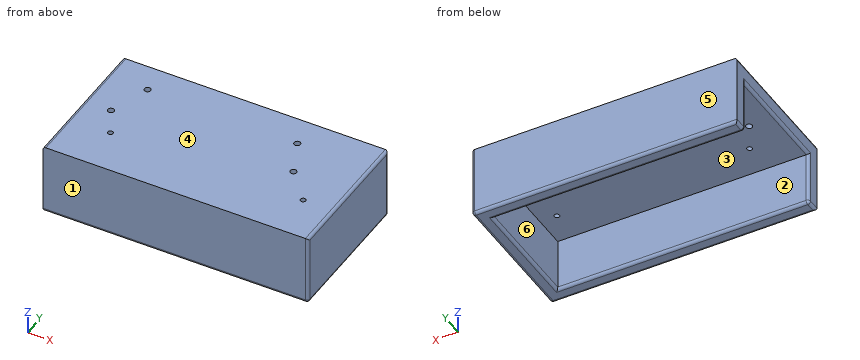
Autodesk Inventor part; units mm, degrees
ref_plane "YZ Plane" through (0, 0, 0) normal (1, 0, 0) x (0, 1, 0)
ref_plane "XZ Plane" through (0, 0, 0) normal (0, 1, 0) x (-1, 0, 0)
ref_plane "XY Plane" through (0, 0, 0) normal (0, 0, 1) x (1, 0, 0)
sketch "스케치1" plane through (0, 0, 0) normal (0, 0, 1) x (1, 0, 0)
  line L0 (-50.4495, 22.5) -> (42.4495, 22.5)
  line L1 (42.4495, 22.5) -> (42.4495, -27.5)
  line L2 (42.4495, -27.5) -> (-50.4495, -27.5)
  line L3 (-50.4495, -27.5) -> (-50.4495, 22.5)
  line L4 (-50.4495, 17.5) -> (37.5505, 17.5)
  line L5 (37.5505, 17.5) -> (37.5505, -22.5)
  line L6 (37.5505, -22.5) -> (-50.4495, -22.5)
  point P0 (0, 0)
  dimension "d0" = 40
  dimension "d1" = 88
  dimension "d2" = 5
  dimension "d3" = 5
extrude "돌출1" add sketch "스케치1" against normal blind 6.2 contours L4 L5 L6 L3
extrude "돌출2" add sketch "스케치1" against normal blind 25 contours L0 L1 L2 L3 L6 L5 L4
sketch "스케치2" plane through (0, 0, -6.2) normal (0, 0, -1) x (-1, 0, 0)
  circle A0 centre (36.2565, 12.6083) radius 1.1
  circle A1 centre (-16.5389, 11.9083) radius 1.1
  circle A2 centre (41.0611, -1.7917) radius 1.1
  circle A3 centre (-22.2389, -0.6917) radius 1.1
  circle A4 centre (35.8561, -11.3917) radius 0.9
  circle A5 centre (-31.6439, -11.3917) radius 0.9
  point P0 (0, 0)
  dimension "d8" = 52.8
  dimension "d9" = 2.2
  dimension "d10" = 2.2
  dimension "d11" = 2.2
  dimension "d12" = 2.2
  dimension "d13" = 63.3
  dimension "d14" = 14.4
  dimension "d15" = 12.6
  dimension "d16" = 1.8
  dimension "d17" = 1.8
  dimension "d18" = 67.5
  dimension "d19" = 10.7
  dimension "d23" = 9.405
  dimension "d24" = 0
  dimension "d25" = 0.7
  dimension "d26" = 5.7
extrude "돌출3" cut sketch "스케치2" against normal blind 63.3
sketch "스케치3" plane through (42.4495, -27.5, 0) normal (1, 0, 0) x (0, 0, -1)
  line L0 (-14.75, 0) -> (-14.75, 50)
  line L1 (-14.75, 50) -> (39.75, 50)
  line L2 (39.75, 50) -> (39.75, 0)
  line L3 (39.75, 0) -> (-14.75, 0)
  line L4 (0, 0) -> (0, 50)
  line L5 (-9.15, 0) -> (-9.15, 50)
  line L6 (34.15, 0) -> (34.15, 50)
  point P0 (0, 27.5)
  dimension "d27" = 54.5
  dimension "d28" = 14.75
  dimension "d29" = 5.6
  dimension "d30" = 43.3
extrude "돌출4" add sketch "스케치3" along normal blind 10
extrude "돌출5" add sketch "스케치3" along normal blind 80 contours L0 L1 L5 L3 | L6 L1 L2 L3
sketch "스케치4" plane through (42.4495, -27.5, 14.75) normal (0, 0, 1) x (1, 0, 0)
  circle A0 centre (25, 27.5) radius 3.75
  line L0 (0, 50) -> (0, 0)
  point P0 (-42.4495, 27.5)
  dimension "d35" = 7.5
  dimension "d36" = 25
extrude "돌출6" cut sketch "스케치4" against normal blind 80
ref_plane "작업 평면1" through (42.4495, -27.5, 0) normal (-1, 0, 0) x (0, 0, 1)
split "분할1" plane through (42.4495, -27.5, 0) removes the side toward (1, 0, 0)
sketch "스케치5" plane through (42.4495, -27.5, 0) normal (1, 0, 0) x (0, 0, -1)
  point P0 (0, 27.5)
sketch "스케치6" plane through (42.4495, -27.5, 0) normal (1, 0, 0) x (0, 0, -1)
  point P0 (0, 27.5)
fillet "모깎기2" radius 1 15 edges at (-6.4495, -22.5, -25) (37.5505, -2.5, -25) (-6.4495, 17.5, -25) (-4, 22.5, -25) (-50.4495, 20, -25) (-50.4495, -25, -25) (-4, -27.5, -25) (42.4495, -2.5, -25) (42.4495, -2.5, 0) (-50.4495, -2.5, 0) (-50.4495, -2.5, -6.2) (-50.4495, 17.5, -15.6) (-50.4495, -22.5, -15.6) (42.4495, 22.5, -12.5) (42.4495, -27.5, -12.5)
equation "\"d21\" = d13"
properties part number "Camera Housing Camera2"
Check sheet for the modelled part. Datum: model origin and axes. Units: mm. Face numbers are marked on the shaded views. A direction names the side the tool comes from. Give positions to 0.01 mm unless a question says otherwise; leave off trailing zeros. Write each loop counter-clockwise with the first axis right and the second up, starting at its lowest first coordinate (ties: lowest second). Pieces come first, ordered by that corner, then holes. Notation, with made-up numbers: M 17,-13 L 45,-13 A18 cw 45,8 Z; hole C 14,-20.75 d5. An arc over 180 degrees is marked long. Use one line per item in the form item = value.
(1) Section check C-C on y = -19. Record the boundary of the cut face in (x, z), plus the area to 3 significant figures.
Answer block:
outline = M -50.45,-5.2 A1 ccw -49.45,-6.2 L 37.55,-6.2 L 37.55,-24 A1 ccw 38.55,-25 L 41.45,-25 A1 ccw 42.45,-24 L 42.45,-1 A1 ccw 41.45,0 L -49.45,0 A1 ccw -50.45,-1 Z
area = 667 mm2
(2) Tool access check on the marked faces 5 and 6. Record the directions out of +Z, -Z, +X, -X, +Y, -Y that give a thin tool (end or side, any length) a straight path to the whole face; none if there is none.
Answer block:
face_5 = +Z, -Z, +X, -X, +Y
face_6 = -Z, -X
(3) Section check B-B on x = -24. Record the boundary of the cut face in (y, z), plus the area to 3 significant figures.
Answer block:
outline = M -27.5,-24 A1 ccw -26.5,-25 L -23.5,-25 A1 ccw -22.5,-24 L -22.5,-6.2 L 17.5,-6.2 L 17.5,-24 A1 ccw 18.5,-25 L 21.5,-25 A1 ccw 22.5,-24 L 22.5,0 L -27.5,0 Z
area = 497 mm2
(4) Draft check along Y on the marked faces 1, 2, 3 and 4. Enter one of: pulls with the +Y half, pulls with the -Y half, needs draft (parallel to the pull), parting line crosses it, or undercut.
Answer block:
face_1 = pulls with the -Y half
face_2 = undercut
face_3 = undercut
face_4 = needs draft
(5) Section check A-A on z = -22.75. Record the boundary of the cut face in (x, y).
Answer block:
outline = M -50.45,-27.5 L 41.45,-27.5 A1 ccw 42.45,-26.5 L 42.45,21.5 A1 ccw 41.45,22.5 L -50.45,22.5 L -50.45,18.5 A1 ccw -49.45,17.5 L 37.55,17.5 L 37.55,-22.5 L -49.45,-22.5 A1 ccw -50.45,-23.5 Z
(6) Material ranges on line 1 along Y through (x, z) = (-8, -10.25); line 2 along X through (y, z) = (-15.5, -23.5); line 3 along Z through (x, y) = (-27.5, -19.5), recorded low to high.
Answer block:
line_1 = -27.5 to -22.5, 17.5 to 22.5
line_2 = 37.55 to 42.45
line_3 = -6.2 to 0
(7) Depth check by flat-ended pin: P1, Ø20, axis at x = 14, y = -11.5, coming from the -Z side; P2, Ø1.4, axis at x = 31.64, y = -11.39, coming from the +Z side; P3, Ø8, axis at y = 7, z = -15, coming from the -X side. Enter the tip coordinate at first touch or a pass-through.
Answer block:
P1 = -6.2
P2 = through
P3 = 37.55
